```python
from build123d import *

# Parameters (mm, degrees)
BOSS_EXTRUDE1_DEPTH = 18.25625
CUT_EXTRUDE1_DEPTH  = 783.681372376
FILLET1_R           = 3.3782


with BuildPart() as part:
    # Sketch1 → Boss-Extrude1 (new body)
    with BuildSketch(Plane(origin=(0, 0, 0), x_dir=(0, 0, -1), z_dir=(1, 0, 0))):
        Polygon((0, 0), (-635, 55.555301339), (-635, -33.3375), (-88.9, -457.2), (0, -457.2), align=None)
    extrude(amount=BOSS_EXTRUDE1_DEPTH)

    # Sketch3 → Cut-Extrude1 (cut, through all)
    with BuildSketch(Plane.ZY):
        Polygon((428.625, -131.7625), (187.325, -319.0875), (152.4, -279.4), (393.7, -92.075), align=None)
    extrude(amount=-CUT_EXTRUDE1_DEPTH, mode=Mode.SUBTRACT)

    # Fillet1
    fillet1_edges = [part.edges().sort_by_distance(p)[0] for p in [
        (9.128125, -319.0875, 187.325),
        (9.128125, -279.4, 152.4),
        (9.128125, -92.075, 393.7),
        (9.128125, -131.7625, 428.625),
    ]]
    fillet(fillet1_edges, radius=FILLET1_R)


solid = part.part
```
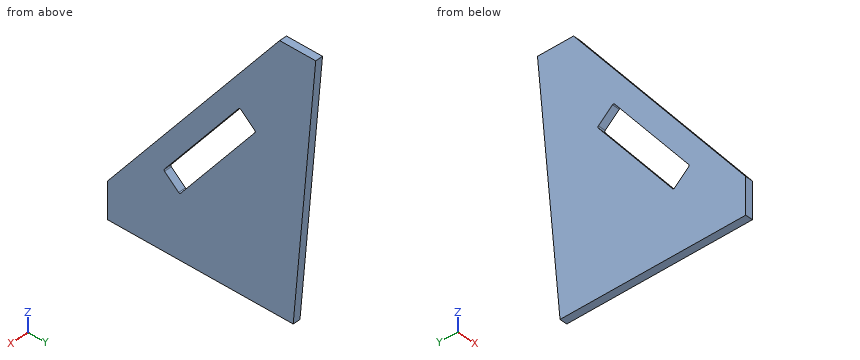
CAD build for the part. Positions are in the model's coordinates, mm. Round coordinates to 2 decimals unless told otherwise and drop trailing zeros. Order: outer loops, then holes, each group sorted by start corner. A loop starts at its lowest first (then second) coordinate and runs counter-clockwise, first axis right, second up.
Item 1: Saw through at A-A on y = -164.5. Write the cut outline in (x, z), then the cut area to 3 significant figures.
Item 2: Saw through at C-C on z = 405.5. Write the cut outline in (x, y), then the cut area to 3 significant figures.
Item 3: Probe line 1 along Z through (x, y) = (10.75, -261); line 2 along Y through (x, z) = (7.5, 310.5); line 3 along Z through (x, y) = (10.25, -231). List the from-to ranges inside material, lowest first.
Item 4: Saw through at D-D on y = -86. Write the cut outline in (x, z).
Item 5: Pin check, flat tips, straight feed: pin 1 (8 mm diameter, centred on x = 14.5, z = 433, fed in from -Y); pin 2 (2 mm diameter, centred on x = 13, y = -110, fed in from +Z); pin 3 (1.5 mm diameter, centred on x = 12.5, y = -216, fed in from +Z). Stop position of each tip, or through.
Item 6: Saw through at B-B on x = 10.25. Write the cut outline in (y, z), then the cut area to 3 significant figures.
Reported:
1. outline: (0, 0) - (18.26, 0) - (18.26, 300.41) - (0, 300.41) - close; (0, 386.45) - (18.26, 386.45) - (18.26, 466.01) - (0, 466.01) - close
1. area: 6,940 mm2
2. outline: (0, -211.47) - (18.26, -211.47) - (18.26, -149.71) - (0, -149.71) - close; (0, -105.48) - (18.26, -105.48) - (18.26, 35.48) - (0, 35.48) - close
2. area: 3,700 mm2
3. line 1: z = 0 to 176.1, 262.15 to 341.68
3. line 2: y = -285.2 to -223.46, -156.66 to 27.17
3. line 3: z = 0 to 214.75, 300.79 to 380.33
4. outline: (0, 0) - (18.26, 0) - (18.26, 567.15) - (0, 567.15) - close
5. pin 1: stops at y = -193.23
5. pin 2: stops at z = 537.52
5. pin 3: stops at z = 400.63
6. outline: (-457.2, 0) - (0, 0) - (55.56, 635) - (-33.34, 635) - (-457.2, 88.9) - close; hole (-317.14, 189.83) arc R3.38 ccw to (-316.7, 185.23) - (-282.1, 154.77) arc R3.38 ccw to (-277.2, 155.24) - (-94.02, 391.19) arc R3.38 ccw to (-94.46, 395.8) - (-129.07, 426.25) arc R3.38 ccw to (-133.97, 425.79) - close
6. area: 176,000 mm2
